```python
from build123d import *

# Parameters (mm, degrees)
SKETCH_1_W          = 98.5
SKETCH_1_H          = 70
EXTRUDE_1_DEPTH     = 5
SKETCH_2_R          = 35
EXTRUDE_2_DEPTH     = 28.1
SKETCH_3_R          = 2
CUT_EXTRUDE_1_DEPTH = 5
FILLET_1_R          = 2
FILLET_2_R          = 1
SKETCH_4_R          = 13
SKETCH_4_W          = 3.316540618
SKETCH_4_H          = 5.120069114
SKETCH_4_W_2        = 3.276095001
SKETCH_4_W_3        = 1.001370982
SKETCH_4_H_2        = 2.121481923
SKETCH_4_H_3        = 2.893302243
SKETCH_4_W_4        = 1.096399653
SKETCH_4_H_4        = 2.99297568
SKETCH_4_W_5        = 1.536933457
SKETCH_4_H_5        = 3.356986235
SKETCH_4_W_6        = 1.658270309
SKETCH_4_W_7        = 1.334705371
SKETCH_4_H_6        = 1.05158605
SKETCH_4_W_8        = 1.294259754
SKETCH_4_H_7        = 1.092031667
CUT_EXTRUDE_3_DEPTH = 0.5
SKETCH_5_R          = 1.25
CUT_EXTRUDE_4_DEPTH = 5
SKETCH_6_R          = 9
EXTRUDE_3_DEPTH     = 7
CUT_EXTRUDE_START   = -1
SKETCH_7_R          = 9
SKETCH_7_R_2        = 0.99350654
CUT_EXTRUDE_5_DEPTH = 1
SKETCH_8_R          = 5.521677929
SKETCH_8_R_2        = 3.001097475
CUT_EXTRUDE_6_DEPTH = 1
FILLET_3_R          = 0.4
SKETCH_9_R          = 16
EXTRUDE_4_DEPTH     = 27
EXTRUDE_5_DEPTH     = 38
SKETCH_11_R         = 26
EXTRUDE_6_DEPTH     = 8
FILLET_4_R          = 1
SKETCH_12_W         = 106.251501727
SKETCH_12_H         = 75.565901032
CUT_EXTRUDE_7_DEPTH = 8
FILLET_5_R          = 100
EXTRUDE_START       = 8
EXTRUDE_7_DEPTH     = 1.6
SKETCH_14_W         = 20
SKETCH_14_H         = 5
EXTRUDE_8_DEPTH     = 6
CHAMFER_1_SIZE      = 1
CUT_EXTRUDE1_START  = -28.1
SKETCH1_R           = 35
CUT_EXTRUDE1_DEPTH  = 28.1


with BuildPart() as part:
    # Эскиз1 → Бобышка-Вытянуть1 (new body)
    with BuildSketch(Plane(origin=(0, 0, 0), x_dir=(1, 0, 0), z_dir=(0, 1, 0))):
        Rectangle(SKETCH_1_W, SKETCH_1_H)
    extrude(amount=EXTRUDE_1_DEPTH)

    # Эскиз2 → Бобышка-Вытянуть2 (add)
    with BuildSketch(Plane(origin=(0, 5, 0), x_dir=(1, 0, 0), z_dir=(0, 1, 0))):
        with Locations(Location((-14.25, 0, 0), (0, 0, 270))):
            Circle(SKETCH_2_R)
    extrude(amount=EXTRUDE_2_DEPTH)

    # Эскиз3 → Вырез-Вытянуть1 (cut)
    with BuildSketch(Plane(origin=(0, 33.1, 0), x_dir=(1, 0, 0), z_dir=(0, 1, 0))):
        with Locations(Location((-14.25, 28.5, 0), (0, 0, 270))):
            Circle(SKETCH_3_R)
        with Locations(Location((-34.553940504, -20, 0), (0, 0, 270))):
            Circle(SKETCH_3_R)
        with Locations(Location((6.053940504, -20, 0), (0, 0, 270))):
            Circle(SKETCH_3_R)
    extrude(amount=-CUT_EXTRUDE_1_DEPTH, mode=Mode.SUBTRACT)

    # Скругление1
    fillet_1_edges = [part.edges().sort_by_distance(p)[0] for p in [
        (-14.25, 33.1, -35),
    ]]
    fillet(fillet_1_edges, radius=FILLET_1_R)

    # Скругление2
    fillet_2_edges = [part.edges().sort_by_distance(p)[0] for p in [
        (-14.25, 33.1, -30.5),
        (-34.553940504, 33.1, 18),
        (6.053940504, 33.1, 18),
    ]]
    fillet(fillet_2_edges, radius=FILLET_2_R)

    # Эскиз4 → Вырез-Вытянуть3 (cut)
    # profile 1 of 7: a face of its own
    with BuildSketch(Plane(origin=(0, 33.1, 0), x_dir=(1, 0, 0), z_dir=(0, 1, 0))):
        with Locations(Location((-14.25, 0, 0), (0, 0, 270))):
            Circle(SKETCH_4_R)
        Polygon((-22.115166942, -6.914876839), (-22.115166942, -0.831627154), (-19.0735421, -0.831627154), (-19.0735421, -5.853844917), (-21.266341405, -5.853844917), (-21.266341405, -6.914876839), align=None, mode=Mode.SUBTRACT)
        Polygon((-22.115166942, 0), (-22.115166942, 5.120069114), (-19.0735421, 5.120069114), (-19.0735421, 4.27071115), (-21.266341405, 4.27071115), (-21.266341405, 0), align=None, mode=Mode.SUBTRACT)
        Polygon((-13.829606569, 0), (-13.829606569, 6.292992015), (-12.980248606, 6.292992015), (-12.980248606, 5.120069114), (-10.715294037, 5.120069114), (-10.715294037, 0), align=None, mode=Mode.SUBTRACT)
        with Locations((-16.458571693, 2.560034557)):
            Rectangle(SKETCH_4_W, SKETCH_4_H, mode=Mode.SUBTRACT)
        with Locations((-8.187442955, 2.560034557)):
            Rectangle(SKETCH_4_W_2, SKETCH_4_H, mode=Mode.SUBTRACT)
        with Locations((-7.050080946, -1.825090787)):
            Rectangle(SKETCH_4_W_3, SKETCH_4_H_2, mode=Mode.SUBTRACT)
        with Locations((-7.050080946, -5.468225718)):
            Rectangle(SKETCH_4_W_3, SKETCH_4_H_3, mode=Mode.SUBTRACT)
        Polygon((-9.825490456, -0.831627154), (-8.643651064, -0.831627154), (-8.643651064, -2.960833634), (-7.550766437, -2.960833634), (-7.550766437, -3.957287265), (-8.643651064, -3.957287265), (-8.643651064, -5.853844917), (-9.825490456, -5.853844917), align=None, mode=Mode.SUBTRACT)
        Polygon((-13.829606569, -0.831627154), (-10.715294037, -0.831627154), (-10.715294037, -5.853844917), (-13.829606569, -5.853844917), (-13.829606569, -3.04994558), (-11.645543235, -3.04994558), (-11.645543235, -1.940786367), (-13.829606569, -1.940786367), align=None, mode=Mode.SUBTRACT)
        Polygon((-18.116842002, -0.831627154), (-14.800301384, -0.831627154), (-14.800301384, -4.141977247), (-16.943919101, -4.141977247), (-16.943919101, -4.950889593), (-14.800301384, -4.950889593), (-14.800301384, -5.853844917), (-18.116842002, -5.853844917), align=None, mode=Mode.SUBTRACT)
    # profile 2 of 7: a face of its own
    with BuildSketch(Plane(origin=(0, 33.1, 0), x_dir=(1, 0, 0), z_dir=(0, 1, 0))):
        with Locations((-20.718141579, -3.454401753)):
            Rectangle(SKETCH_4_W_4, SKETCH_4_H_4)
    # profile 3 of 7: a face of its own
    with BuildSketch(Plane(origin=(0, 33.1, 0), x_dir=(1, 0, 0), z_dir=(0, 1, 0))):
        with Locations((-8.167220148, 2.592218033)):
            Rectangle(SKETCH_4_W_5, SKETCH_4_H_5)
    # profile 4 of 7: a face of its own
    with BuildSketch(Plane(origin=(0, 33.1, 0), x_dir=(1, 0, 0), z_dir=(0, 1, 0))):
        with Locations((-16.478794502, 2.592218033)):
            Rectangle(SKETCH_4_W_6, SKETCH_4_H_5)
    # profile 5 of 7: a face of its own
    with BuildSketch(Plane(origin=(0, 33.1, 0), x_dir=(1, 0, 0), z_dir=(0, 1, 0))):
        with Locations((-12.312895921, 2.592218033)):
            Rectangle(SKETCH_4_W_7, SKETCH_4_H_5)
    # profile 6 of 7: a face of its own
    with BuildSketch(Plane(origin=(0, 33.1, 0), x_dir=(1, 0, 0), z_dir=(0, 1, 0))):
        with Locations((-12.312895921, -4.667770272)):
            Rectangle(SKETCH_4_W_7, SKETCH_4_H_6)
    # profile 7 of 7: a face of its own
    with BuildSketch(Plane(origin=(0, 33.1, 0), x_dir=(1, 0, 0), z_dir=(0, 1, 0))):
        with Locations((-16.296789224, -2.503929746)):
            Rectangle(SKETCH_4_W_8, SKETCH_4_H_7)
    extrude(amount=-CUT_EXTRUDE_3_DEPTH, mode=Mode.SUBTRACT)

    # Эскиз5 → Вырез-Вытянуть4 (cut)
    with BuildSketch(Plane(origin=(0, 5, 0), x_dir=(1, 0, 0), z_dir=(0, 1, 0))):
        with Locations(Location((-42.25, 28, 0), (0, 0, 270))):
            Circle(SKETCH_5_R)
        with Locations(Location((27.75, 20, 0), (0, 0, 270))):
            Circle(SKETCH_5_R)
        with Locations(Location((27.75, -20, 0), (0, 0, 90))):
            Circle(SKETCH_5_R)
        with Locations(Location((-42.25, -28, 0), (0, 0, 90))):
            Circle(SKETCH_5_R)
    extrude(amount=-CUT_EXTRUDE_4_DEPTH, mode=Mode.SUBTRACT)

    # Эскиз6 → Бобышка-Вытянуть3 (add)
    with BuildSketch(Plane(origin=(0, 5, 0), x_dir=(1, 0, 0), z_dir=(0, 1, 0))):
        with Locations(Location((31.25, 0, 0), (0, 0, 270))):
            Circle(SKETCH_6_R)
    extrude(amount=EXTRUDE_3_DEPTH)

    # Эскиз7 → Вырез-Вытянуть5 (cut)
    with BuildSketch(Plane(origin=(0, 12, 0), x_dir=(1, 0, 0), z_dir=(0, 1, 0)).offset(CUT_EXTRUDE_START)):
        with Locations(Location((31.25, 0, 0), (0, 0, 270))):
            Circle(SKETCH_7_R)
        with Locations(Location((31.25, 0, 0), (0, 0, 270))):
            Circle(SKETCH_7_R_2, mode=Mode.SUBTRACT)
    extrude(amount=CUT_EXTRUDE_5_DEPTH, mode=Mode.SUBTRACT)

    # Эскиз8 → Вырез-Вытянуть6 (cut)
    with BuildSketch(Plane(origin=(0, 11, 0), x_dir=(1, 0, 0), z_dir=(0, 1, 0))):
        with Locations(Location((31.25, 0, 0), (0, 0, 270))):
            Circle(SKETCH_8_R)
        with Locations(Location((31.25, 0, 0), (0, 0, 270))):
            Circle(SKETCH_8_R_2, mode=Mode.SUBTRACT)
    extrude(amount=-CUT_EXTRUDE_6_DEPTH, mode=Mode.SUBTRACT)

    # Скругление3
    fillet_3_edges = [part.edges().sort_by_distance(p)[0] for p in [
        (31.25, 12, -0.99350654),
    ]]
    fillet(fillet_3_edges, radius=FILLET_3_R)

    # Эскиз9 → Бобышка-Вытянуть4 (add)
    with BuildSketch(Plane(origin=(0, 5, 0), x_dir=(1, 0, 0), z_dir=(0, 1, 0))):
        with Locations(Location((31.25, 0, 0), (0, 0, 270))):
            Circle(SKETCH_9_R)
    extrude(amount=-EXTRUDE_4_DEPTH)

    # Эскиз10 → Бобышка-Вытянуть5 (add)
    with BuildSketch(Plane.XZ):
        Polygon((-40.854614908, 25.472900125), (-39.363774764, 27.944889), (-40.759159856, 30.471988875), (-43.645385092, 30.527099875), (-45.136225236, 28.055111), (-43.740840144, 25.528011125), align=None)
        Polygon((29.257133708, 22.462088812), (26.371335397, 22.536260484), (24.864201688, 20.074171672), (26.242866292, 17.537911188), (29.128664603, 17.463739516), (30.635798312, 19.925828328), align=None)
        Polygon((30.635798312, -19.925828328), (29.257133708, -22.462088812), (26.371335397, -22.536260484), (24.864201688, -20.074171672), (26.242866292, -17.537911188), (29.128664603, -17.463739516), align=None)
        Polygon((-43.740840144, -25.528011125), (-40.854614908, -25.472900125), (-39.363774764, -27.944889), (-40.759159856, -30.471988875), (-43.645385092, -30.527099875), (-45.136225236, -28.055111), align=None)
    extrude(amount=EXTRUDE_5_DEPTH)

    # Эскиз11 → Бобышка-Вытянуть6 (add)
    with BuildSketch(Plane(origin=(0, 5, 0), x_dir=(1, 0, 0), z_dir=(0, 1, 0))):
        with Locations(Location((-14.25, 0, 0), (0, 0, 270))):
            Circle(SKETCH_11_R)
    extrude(amount=-EXTRUDE_6_DEPTH)

    # Скругление4
    fillet_4_edges = [part.edges().sort_by_distance(p)[0] for p in [
        (-14.25, -3, -26),
    ]]
    fillet(fillet_4_edges, radius=FILLET_4_R)

    # Эскиз12 → Вырез-Вытянуть7 (cut)
    with BuildSketch(Plane(origin=(0, 5, 0), x_dir=(1, 0, 0), z_dir=(0, 1, 0))):
        with Locations((-0.925367694, -0.052186396)):
            Rectangle(SKETCH_12_W, SKETCH_12_H)
        with BuildLine():
            ThreePointArc((-49.25, 0), (-48.116981176, 14.083966884), (-45.528607092, 27.974329531))
            ThreePointArc((-45.528607092, 27.974329531), (-44.561596332, 29.769996926), (-42.834972324, 30.855492545))
            ThreePointArc((-42.834972324, 30.855492545), (2.249574036, 33.221442581), (42.908955543, 13.599293477))
            ThreePointArc((42.908955543, 13.599293477), (47.577997957, 7.498372972), (49.25, 0))
            ThreePointArc((49.25, 0), (47.577997957, -7.498372972), (42.908955543, -13.599293477))
            ThreePointArc((42.908955543, -13.599293477), (2.249574036, -33.221442581), (-42.834972324, -30.855492545))
            ThreePointArc((-42.834972324, -30.855492545), (-44.561596332, -29.769996926), (-45.528607092, -27.974329531))
            ThreePointArc((-45.528607092, -27.974329531), (-48.116981176, -14.083966884), (-49.25, 0))
        make_face(mode=Mode.SUBTRACT)
    extrude(amount=-CUT_EXTRUDE_7_DEPTH, mode=Mode.SUBTRACT)

    # Скругление5
    # the kernel refuses this fillet: 100 mm, written as the material it takes off along each edge
    with BuildSketch(Plane(origin=(-49.25, 5, 0), x_dir=(0.06766370453174418, 0, 0.9977081853372963), z_dir=(0, -1, 0))) as fillet_5_piece_1:
        with BuildLine():
            CenterArc((6.776645039, -99.922318338), FILLET_5_R, 87.741474483, 12.276669201)
            ThreePointArc((-10.619357471, -1.44704684), (-5.323940761, -0.618859533), (0, 0))
            ThreePointArc((0, 0), (5.358747467, 0.105631125), (10.717494933, 0))
        make_face()
    extrude(amount=31.793737334, mode=Mode.SUBTRACT)

    # Эскиз13 → Бобышка-Вытянуть7 (add)
    with BuildSketch(Plane.XZ.offset(EXTRUDE_START)):
        with BuildLine():
            Line((31.553634402, 21.860321538), (31.553634402, 16.4))
            ThreePointArc((31.553634402, 16.4), (15.153634402, 0), (31.553634402, -16.4))
            Line((31.553634402, -16.4), (31.553634402, -21.860321538))
            ThreePointArc((31.553634402, -21.860321538), (-4.596615235, -34.347840749), (-42.683124513, -30.855492545))
            ThreePointArc((-42.683124513, -30.855492545), (-44.409748521, -29.769996926), (-45.37675928, -27.974329531))
            ThreePointArc((-45.37675928, -27.974329531), (-47.965133365, -14.083966884), (-49.098152188, 0))
            ThreePointArc((-49.098152188, 0), (-47.965133365, 14.083966884), (-45.37675928, 27.974329531))
            ThreePointArc((-45.37675928, 27.974329531), (-44.409748521, 29.769996926), (-42.683124513, 30.855492545))
            ThreePointArc((-42.683124513, 30.855492545), (-4.596615235, 34.347840749), (31.553634402, 21.860321538))
        make_face()
    extrude(amount=EXTRUDE_7_DEPTH)

    # Эскиз14 → Бобышка-Вытянуть8 (add)
    with BuildSketch(Plane.XZ.offset(9.6)):
        with Locations((-14.098152188, 27.5)):
            Rectangle(SKETCH_14_W, SKETCH_14_H)
    extrude(amount=EXTRUDE_8_DEPTH)

    # Фаска1
    chamfer_1_edges = [part.edges().sort_by_distance(p)[0] for p in [
        (-24.098152188, -12.6, 30),
    ]]
    chamfer(chamfer_1_edges, length=CHAMFER_1_SIZE)

    # Sketch1 → Cut-Extrude1 (cut)
    with BuildSketch(Plane(origin=(0, 33.1, 0), x_dir=(1, 0, 0), z_dir=(0, 1, 0)).offset(CUT_EXTRUDE1_START)):
        with Locations((-14.25, 0)):
            Circle(SKETCH1_R)
    extrude(amount=CUT_EXTRUDE1_DEPTH, mode=Mode.SUBTRACT)


solid = part.part
```
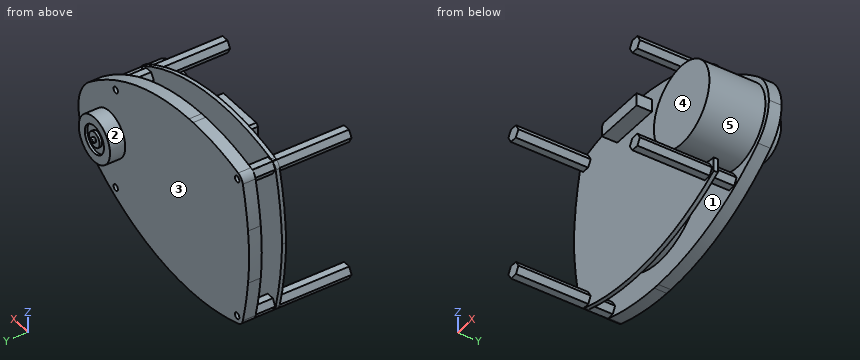
Can you work these out from the model? Positions are in its coordinate system, mm. Face numbers are marked on the shaded views. A direction names the side the tool comes from. Coordinates: 2 decimals unless noted, no trailing zeros. Write each loop counter-clockwise with the first axis right and the second up, starting at its lowest first coordinate (ties: lowest second). Pieces come first, ordered by that corner, then holes. Notation, with made-up numbers: M 74,-25.75 L 120,-25.75 A18 ccw 120,5.25 Z; hole C 46,-11.5 d8. An arc over 180 degrees is marked long. Write item = value, one per line. Start each with the question number.
Q1. If I drill on L1, parallel to X at y = 10.7, z = 0; L2, parallel to Y at x = -5.5, z = 2; L3, parallel to Z at x = 25.5, y = -17, over which ranges is the centre line in solid material (lowest first)? Write a range as [from, to].
Q2. Thinking about a two-plate mould opening in Z: for the marked faces 1, 2 and 3, which applies, released by +Z, released by -Z, zero draft, split by the parting line, or undercut?
Q3. On a 3-axis mill with a long thin cutter (end or side, diameter ignored), from which of +Z, -Z, +X, -X, +Y, -Y can I reach the whole of each face in a straight line? I mean the marked faces 4 and 5. Say none if no direction works.
Q4. If we section it at A-A, the plane y = -35: Write out the boundary of the cut face in (x, z), then the cut area to 3 significant figures.
Q5. If we section it at B-B, the plane y = 2: Write out the boundary of the cut face in (x, z), then the cut area to 3 significant figures.
Q6. I'm going to push flat-ended pins straight in: pin 1 (5 mm diameter, centred on x = 30, y = -26, fed in from -Z); pin 2 (0.7 mm diameter, centred on x = -15.5, y = 2.5, fed in from +Z); pin 3 (2 mm diameter, centred on y = 4, z = 5.5, fed in from +X). Where does each tip first touch, or does it pass through?
Check sheet entries:
q1.L1 = [22.25, 25.73], [28.25, 34.25], [36.77, 40.25]
q1.L2 = [-9.6, -8], [-3, 5]
q1.L3 = [-21.11, -18.9], [-14.93, 14.93], [18.9, 21.11]
q2.face_1 = undercut
q2.face_2 = split by the parting line
q2.face_3 = zero draft
q3.face_4 = +X, -X, -Y
q3.face_5 = -Y
q4.outline = M -45.14,-28.06 L -43.65,-30.53 L -40.76,-30.47 L -39.36,-27.94 L -40.85,-25.47 L -43.74,-25.53 Z; M -45.14,28.06 L -43.74,25.53 L -40.85,25.47 L -39.36,27.94 L -40.76,30.47 L -43.65,30.53 Z; M 24.86,-20.07 L 26.37,-22.54 L 29.26,-22.46 L 30.64,-19.93 L 29.13,-17.46 L 26.24,-17.54 Z; M 24.86,20.07 L 26.24,17.54 L 29.13,17.46 L 30.64,19.93 L 29.26,22.46 L 26.37,22.54 Z
q4.area = 86.6 mm²
q5.outline = M -48.52,-10.69 A135.98 ccw -45.53,-27.97 A4 ccw -42.83,-30.86 A90.87 ccw -16.86,-35 L -14.5,-35 A90.87 ccw 42.91,-13.6 A17.85 ccw 49.25,0 A17.85 ccw 42.91,13.6 A90.87 ccw -14.5,35 L -16.86,35 A90.87 ccw -42.83,30.86 A4 ccw -45.53,27.97 A135.98 ccw -48.52,10.69 A100 ccw Z; hole C -42.25,-28 d2.5; hole C -42.25,28 d2.5; hole C 27.75,-20 d2.5; hole C 27.75,20 d2.5
q5.area = 5,530 mm²
q6.pin_1 = -22.51
q6.pin_2 = 35
q6.pin_3 = 48.66
